Geometry check sheet. Reference: drawing and pictorial views, mm from the part's lowest x, y, z. A direction names the side the tool comes from. Give positions to 0.01 mm unless a question says otherwise; leave off trailing zeros. Loops run counter-clockwise (first coordinate to the right, second up) from the corner with the lowest first, then second, coordinate; pieces in that order, holes last. Notation, with made-up numbers: M -39.75,13 L -12.75,13 A32 ccw -12.75,41 Z; hole C 89.5,-31 d6. An arc over 180 degrees is marked long. Put each result on its own line as item: value. Start each with the question number.
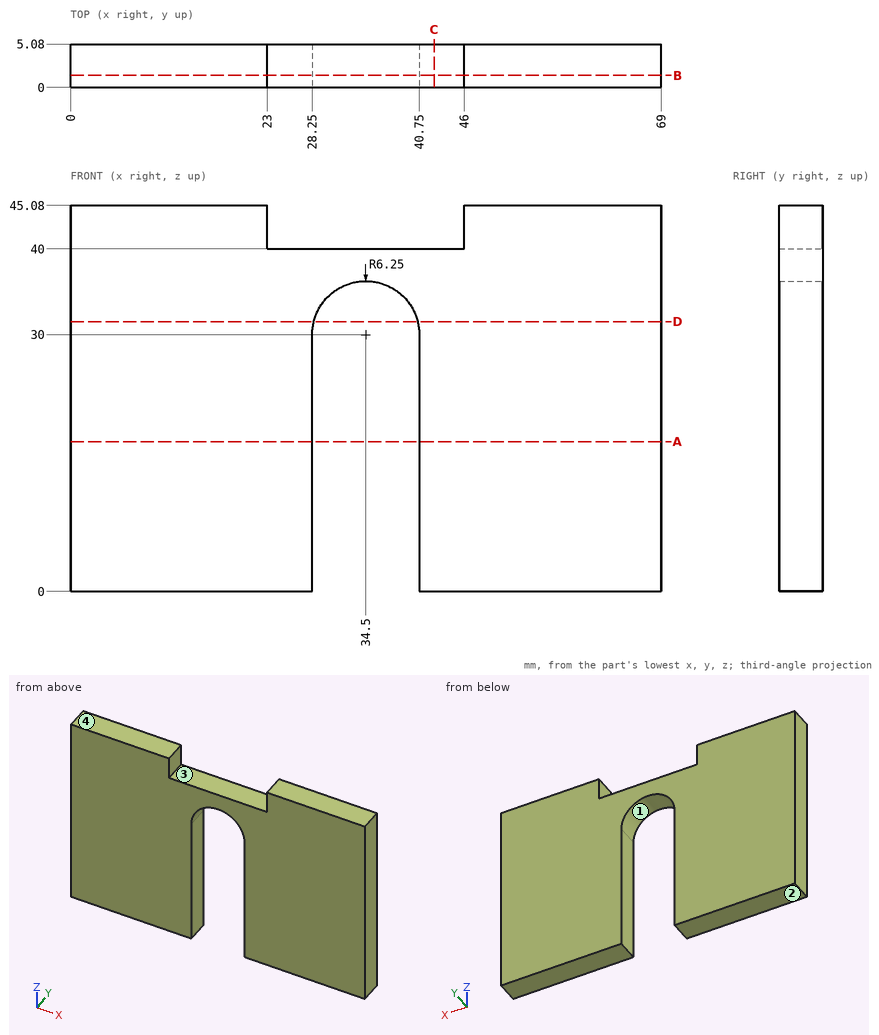
Q1. Mould release check, pull along X, two halves, no side actions. Record for the marked faces 1 and 2: pulls with the +X half, pulls with the -X half, needs draft (parallel to the pull), parting line crosses it, or undercut.
Q2. Depth check by flat-ended pin: P1, Ø2, axis at x = 33.5, y = 2.5, coming from the +Z side. Enter the tip coordinate at first touch or a pass-through.
Q3. Access from +Z, -Z, +X, -X, +Y, -Y to the whole of each face (thin tool, end or side, straight path). Record for the marked faces 3 and 4.
Q4. Section check A-A, the plane z = 17.5. Record the cut outline in (x, y).
Q5. Section check C-C, the plane x = 42.5. Record the cut outline in (y, z), then the cut area to 3 significant figures.
Q6. Thickness scan on line 1 along X through (y, z) = (0.35, 19); line 2 along X through (y, z) = (2.3, 31); line 3 along Z through (x, y) = (45, 2.1). Record the ranges inside material, lowest first. Write a range as [from, to].
Q7. Section check B-B, the plane y = 1.4. Record the cut outline in (x, z), then the cut area to 3 significant figures.
Q8. Section check D-D, the plane z = 31.5. Record the cut outline in (x, y), then the cut area to 3 significant figures.
Found:
1. face 1: undercut
1. face 2: needs draft
2. P1: stops at z = 40
3. face 3: +Z, +Y, -Y
3. face 4: +Z, +X, -X, +Y, -Y
4. outline: M 0,0 L 28.25,0 L 28.25,5.08 L 0,5.08 Z; M 40.75,0 L 69,0 L 69,5.08 L 40.75,5.08 Z
5. outline: M 0,0 L 5.08,0 L 5.08,40 L 0,40 Z
5. area: 203 mm^2
6. line 1: x = [0, 28.25], [40.75, 69]
6. line 2: x = [0, 28.33], [40.67, 69]
6. line 3: z = [0, 40]
7. outline: M 0,0 L 28.25,0 L 28.25,30 A6.25 cw 40.75,30 L 40.75,0 L 69,0 L 69,45.08 L 46,45.08 L 46,40 L 23,40 L 23,45.08 L 0,45.08 Z
7. area: 2,560 mm^2
8. outline: M 0,0 L 28.43,0 L 28.43,5.08 L 0,5.08 Z; M 40.57,0 L 69,0 L 69,5.08 L 40.57,5.08 Z
8. area: 289 mm^2
